Geometry: final body of the model. Coordinates: model frame, mm. A direction names the side the tool comes from. Give positions to 0.01 mm unless a question says otherwise; leave off trailing zeros. Write each loop counter-clockwise with the first axis right and the second up, starting at its lowest first coordinate (ties: lowest second). Pieces come first, ordered by that corner, then holes. Notation, with made-up numbers: (60.5, 66.5) - (87.5, 66.5) arc R25 cw to (87.5, 101.5) - close; hole circle Ø3 at (72, 43). An arc over 180 degrees is marked (long way). Return JSON: item names as keys, results as strings.
from build123d import *

# Parameters (mm, degrees)
SKETCH1_R           = 1.25
BOSS_EXTRUDE1_DEPTH = 2
SKETCH2_W           = 1.8
SKETCH2_H           = 2.8
SKETCH2_W_2         = 2
SKETCH2_H_2         = 5
BOSS_EXTRUDE2_DEPTH = 4


with BuildPart() as part:
    # Sketch1 → Boss-Extrude1 (new body)
    with BuildSketch(Plane.XY):
        with BuildLine():
            Line((-14.5, -1.25), (-3.25, -1.25))
            Line((-3.25, -1.25), (-3.25, 0))
            ThreePointArc((-3.25, 0), (0, 3.25), (3.25, 0))
            Line((3.25, 0), (3.25, -1.25))
            Line((3.25, -1.25), (7.5, -1.25))
            ThreePointArc((7.5, -1.25), (10, -3.75), (7.5, -6.25))
            Line((7.5, -6.25), (-14.5, -6.25))
            ThreePointArc((-14.5, -6.25), (-17, -3.75), (-14.5, -1.25))
        make_face()
        Circle(SKETCH1_R, mode=Mode.SUBTRACT)
    extrude(amount=BOSS_EXTRUDE1_DEPTH)

    # Sketch2 → Boss-Extrude2 (add)
    with BuildSketch(Plane.XY.offset(2)):
        with Locations((-2.1, -4.85)):
            Rectangle(SKETCH2_W, SKETCH2_H)
        with Locations((2.1, -4.85)):
            Rectangle(SKETCH2_W, SKETCH2_H)
        with Locations((-9, -3.75)):
            Rectangle(SKETCH2_W_2, SKETCH2_H_2)
        with BuildLine():
            ThreePointArc((8, -6.199489743), (10, -3.75), (8, -1.300510257))
            Line((8, -1.300510257), (8, -6.199489743))
        make_face()
        with BuildLine():
            Line((-15, -6.199489743), (-15, -1.300510257))
            ThreePointArc((-15, -1.300510257), (-17, -3.75), (-15, -6.199489743))
        make_face()
    extrude(amount=BOSS_EXTRUDE2_DEPTH)


solid = part.part
Q1. Pin query (flat end, axial travel): P1, Ø1.2, axis at y = -3, z = 4.5, coming from the +X side; P2, Ø1.2, axis at y = -5, z = 4, coming from the -X side; P3, Ø2, axis at x = 2, z = 3.5, coming from the +Y side. Return the tip coordinate at first contact, or that it passes through.
Answer key:
{"P1": "stops at x = 10", "P2": "stops at x = -16.91", "P3": "stops at y = -3.45"}
Q2. Set-up query: faces 1 (the flat face through (-9, -1.25, 2)), 2 (the flat face through (-2, -3.45, 4)), 3 (the flat face through (5, -1.25, 1)), 4 (the flat face through (-8, -4, 4)). Return all of +Z, -Z, +X, -X, +Y, -Y with unobstructed straight access to the full face (end or side cutting, diameter ignored); none if empty.
Answer key:
{"face 1": "+Z, -Z, -X, +Y", "face 2": "+Z, +Y", "face 3": "+Z, -Z, +X, +Y", "face 4": "+Z, +Y, -Y"}
Q3. Section query C-C, the plane x = 0. Return the cut outline in (y, z), plus the area to 3 significant figures.
Answer key:
{"outline": "(-6.25, 0) - (-1.25, 0) - (-1.25, 2) - (-6.25, 2) - close; (1.25, 0) - (3.25, 0) - (3.25, 2) - (1.25, 2) - close", "area": "14.0 mm^2"}
Q4. Section query D-D, the plane y = 1. Return the cut outline in (x, z), plus the area to 3 significant figures.
Answer key:
{"outline": "(-3.09, 0) - (-0.75, 0) - (-0.75, 2) - (-3.09, 2) - close; (0.75, 0) - (3.09, 0) - (3.09, 2) - (0.75, 2) - close", "area": "9.37 mm^2"}
Q5. Section query A-A, the plane z = 2.3. Return the cut outline in (x, y).
Answer key:
{"outline": "(-15, -6.2) - (-15, -1.3) arc R2.5 ccw to start; (-10, -6.25) - (-8, -6.25) - (-8, -1.25) - (-10, -1.25) - close; (-3, -6.25) - (-1.2, -6.25) - (-1.2, -3.45) - (-3, -3.45) - close; (1.2, -6.25) - (3, -6.25) - (3, -3.45) - (1.2, -3.45) - close; (8, -6.2) arc R2.5 ccw to (8, -1.3) - close"}
Q6. Section query B-B, the plane z = 1.2. Return the cut outline in (x, y).
Answer key:
{"outline": "(-14.5, -6.25) - (7.5, -6.25) arc R2.5 ccw to (7.5, -1.25) - (3.25, -1.25) - (3.25, 0) arc R3.25 ccw to (-3.25, 0) - (-3.25, -1.25) - (-14.5, -1.25) arc R2.5 ccw to start; hole circle Ø2.5 at (0, 0)"}
Q7. Material intervals for probe 1 along Y at (x, z) = (0, 0.6); probe 2 along X at (y, z) = (-5.25, 3.85); probe 3 along X at (y, z) = (-1.75, 2.9), sorted ascending. Write a range as [from, to].
Answer key:
{"probe 1": "y = [-6.25, -1.25], [1.25, 3.25]", "probe 2": "x = [-16.5, -15], [-10, -8], [-3, -1.2], [1.2, 3], [8, 9.5]", "probe 3": "x = [-16, -15], [-10, -8], [8, 9]"}
